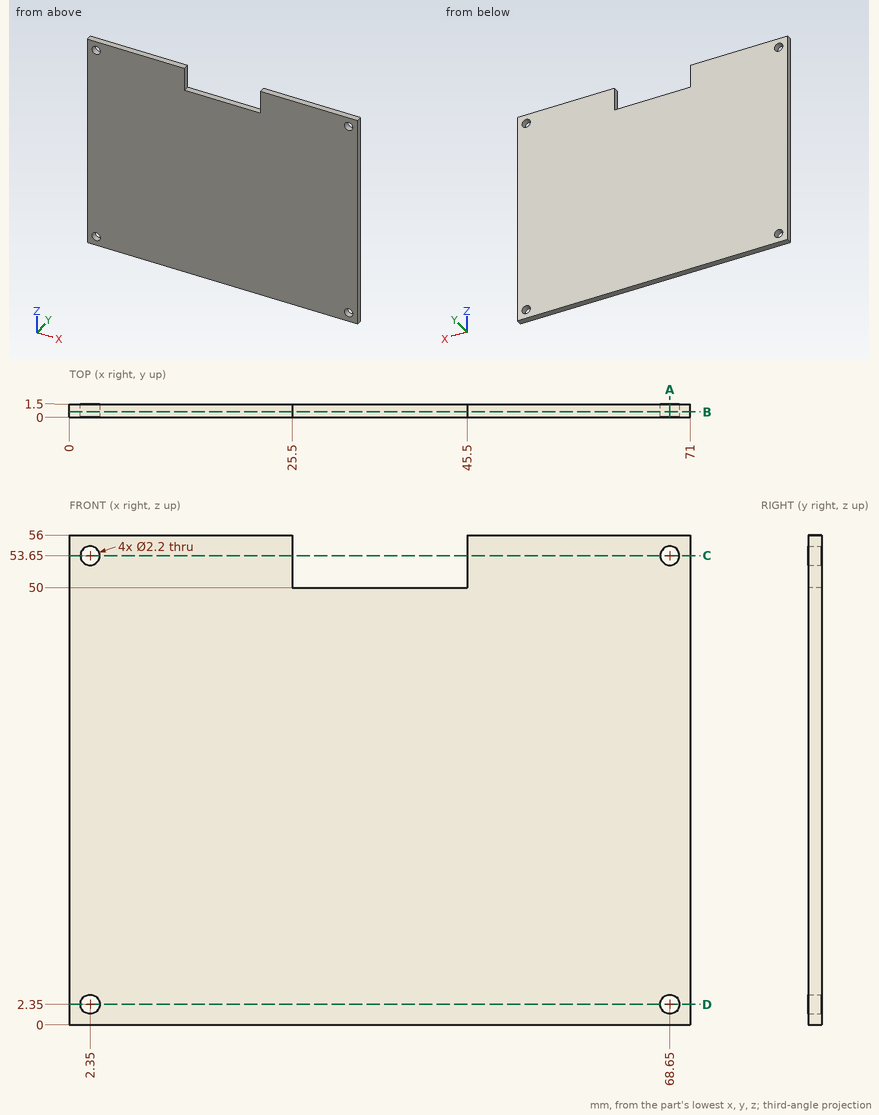
Check sheet for the drawn part. Datum: minimum x, y, z corner. Units: mm. Coordinates: 2 decimals unless noted, no trailing zeros. Order: outer loops, then holes, each group sorted by start corner. A loop starts at its lowest first (then second) coordinate and runs counter-clockwise, first axis right, second up. Notation, with made-up numbers: (-14.75, 84.5) -> (4.25, 84.5) arc R19 cw to (4.25, 113.5) -> close; hole circle Ø10 at (86.25, -15.5). An arc over 180 degrees is marked (long way). Write each question's results on one line, items separated by ' | '. Start each with the question number.
1) Section check B-B (y = 0.6). Enter the section's corners in (x, z), and give its area (3 significant figures).
2) Section check C-C (z = 53.65). Enter the section's corners in (x, y).
3) Section check A-A (x = 68.65). Enter the section's corners in (y, z), and give its area (3 significant figures).
4) Section check D-D (z = 2.35). Enter the section's corners in (x, y).
5) Material ranges on line 1 along Z through (x, y) = (2.35, 1.2); line 2 along Z through (x, y) = (28, 0.4), recorded low to high.
Checked values:
1) outline: (0, 0) -> (71, 0) -> (71, 56) -> (45.5, 56) -> (45.5, 50) -> (25.5, 50) -> (25.5, 56) -> (0, 56) -> close; hole circle Ø2.2 at (2.35, 2.35); hole circle Ø2.2 at (2.35, 53.65); hole circle Ø2.2 at (68.65, 2.35); hole circle Ø2.2 at (68.65, 53.65) | area: 3,840 mm²
2) outline: (0, 0) -> (1.25, 0) -> (1.25, 1.5) -> (0, 1.5) -> close; (3.45, 0) -> (25.5, 0) -> (25.5, 1.5) -> (3.45, 1.5) -> close; (45.5, 0) -> (67.55, 0) -> (67.55, 1.5) -> (45.5, 1.5) -> close; (69.75, 0) -> (71, 0) -> (71, 1.5) -> (69.75, 1.5) -> close
3) outline: (0, 0) -> (1.5, 0) -> (1.5, 1.25) -> (0, 1.25) -> close; (0, 3.45) -> (1.5, 3.45) -> (1.5, 52.55) -> (0, 52.55) -> close; (0, 54.75) -> (1.5, 54.75) -> (1.5, 56) -> (0, 56) -> close | area: 77.4 mm²
4) outline: (0, 0) -> (1.25, 0) -> (1.25, 1.5) -> (0, 1.5) -> close; (3.45, 0) -> (67.55, 0) -> (67.55, 1.5) -> (3.45, 1.5) -> close; (69.75, 0) -> (71, 0) -> (71, 1.5) -> (69.75, 1.5) -> close
5) line 1: 0 to 1.25, 3.45 to 52.55, 54.75 to 56 | line 2: 0 to 50
